Work out the finished part from the listing and answer in its coordinate system (mm). A direction names the side the tool comes from. Give positions to 0.01 mm unless a question says otherwise; leave off trailing zeros. Loops run counter-clockwise (first coordinate to the right, second up) from the corner with the lowest first, then second, coordinate; pieces in that order, holes last. Notation, with made-up numbers: M -6.75,64.5 L -2.75,64.5 A24 ccw -2.75,102.5 Z; hole C 1,19 d7. An arc over 180 degrees is marked long. Use a Markdown table: item, result.
```python
from build123d import *

# Parameters (mm, degrees)
BASE_W              = 40
BASE_H              = 59
EXTRUDE_1_DEPTH     = 2
SKETCH_2_W          = 40
SKETCH_2_H          = 59
SKETCH_2_W_2        = 35
SKETCH_2_H_2        = 54
EXTRUDE_2_DEPTH     = 10
SKETCH_3_R          = 3.25
EXTRUDE_3_DEPTH     = 5
SKETCH_4_R          = 2.9
CUT_EXTRUDE_2_DEPTH = 5
CHAMFER_1_SIZE      = 1.5
CHAMFER_1_SIZE_2    = 5.598076211
SKETCH_6_R          = 1.75
CUT_EXTRUDE_3_DEPTH = 38.896736188
FILLET_1_R          = 5
SKETCH_7_W          = 40
SKETCH_7_H          = 59
SKETCH_7_W_2        = 39
SKETCH_7_H_2        = 58
CUT_EXTRUDE_6_DEPTH = 6
CHAMFER_2_SIZE      = 1
SKETCH_8_W          = 43.293299122
SKETCH_8_H          = 71.249143308
CUT_EXTRUDE_7_DEPTH = 0.1
SKETCH_9_W          = 16
SKETCH_9_H          = 3
CUT_EXTRUDE_8_DEPTH = 64.13297577


with BuildPart() as part:
    # base → Бобышка-Вытянуть1 (new body)
    with BuildSketch(Plane.XY):
        with Locations((-0.540511526, 0)):
            Rectangle(BASE_W, BASE_H)
    extrude(amount=EXTRUDE_1_DEPTH)

    # Эскиз2 → Бобышка-Вытянуть2 (add)
    with BuildSketch(Plane.XY.offset(2)):
        with Locations((-0.540511526, 0)):
            Rectangle(SKETCH_2_W, SKETCH_2_H)
        with Locations((-0.540511526, 0)):
            Rectangle(SKETCH_2_W_2, SKETCH_2_H_2, mode=Mode.SUBTRACT)
    extrude(amount=EXTRUDE_2_DEPTH)

    # Эскиз3 → Бобышка-Вытянуть3 (add)
    with BuildSketch(Plane.XY.offset(2)):
        with Locations((-14.040511526, -23)):
            Circle(SKETCH_3_R)
        with Locations((12.959488474, -23)):
            Circle(SKETCH_3_R)
        with Locations((12.959488474, 23)):
            Circle(SKETCH_3_R)
        with Locations((-14.040511526, 23)):
            Circle(SKETCH_3_R)
    extrude(amount=EXTRUDE_3_DEPTH)

    # Эскиз4 → Вырез-Вытянуть2 (cut)
    with BuildSketch(Plane(origin=(0, 0, 0), x_dir=(-1, 0, 0), z_dir=(0, 0, -1))):
        with Locations((14.040511526, -23)):
            Circle(SKETCH_4_R)
        with Locations((-12.959488474, -23)):
            Circle(SKETCH_4_R)
        with Locations((-12.959488474, 23)):
            Circle(SKETCH_4_R)
        with Locations((14.040511526, 23)):
            Circle(SKETCH_4_R)
    extrude(amount=-CUT_EXTRUDE_2_DEPTH, mode=Mode.SUBTRACT)

    # Фаска1
    # the kernel refuses this chamfer: 5.598076211, 1.5 mm, written as the material it adds along each edge
    with BuildSketch(Plane(origin=(-14.040511526, 23, 2), x_dir=(1, 0, 0), z_dir=(0, -1, 0))) as chamfer_1_piece_1_section:
        Polygon((3.25 + CHAMFER_1_SIZE, 0), (3.25, CHAMFER_1_SIZE_2), (3.25, 0), align=None)
    chamfer_1_piece_1 = revolve(axis=Axis((-14.040511526, 23, 2), (0, 0, 1)), mode=Mode.PRIVATE)
    chamfer_1_piece_1 = split(chamfer_1_piece_1, bisect_by=Plane(origin=(-14.040511526, 23, 7), z_dir=(0, 0, -1)), keep=Keep.TOP, mode=Mode.PRIVATE)
    add(chamfer_1_piece_1)
    with BuildSketch(Plane(origin=(12.959488474, 23, 2), x_dir=(1, 0, 0), z_dir=(0, -1, 0))) as chamfer_1_piece_2_section:
        Polygon((3.25 + CHAMFER_1_SIZE, 0), (3.25, CHAMFER_1_SIZE_2), (3.25, 0), align=None)
    chamfer_1_piece_2 = revolve(axis=Axis((12.959488474, 23, 2), (0, 0, 1)), mode=Mode.PRIVATE)
    chamfer_1_piece_2 = split(chamfer_1_piece_2, bisect_by=Plane(origin=(12.959488474, 23, 7), z_dir=(0, 0, -1)), keep=Keep.TOP, mode=Mode.PRIVATE)
    add(chamfer_1_piece_2)
    with BuildSketch(Plane(origin=(-14.040511526, -23, 2), x_dir=(1, 0, 0), z_dir=(0, -1, 0))) as chamfer_1_piece_3_section:
        Polygon((3.25 + CHAMFER_1_SIZE, 0), (3.25, CHAMFER_1_SIZE_2), (3.25, 0), align=None)
    chamfer_1_piece_3 = revolve(axis=Axis((-14.040511526, -23, 2), (0, 0, 1)), mode=Mode.PRIVATE)
    chamfer_1_piece_3 = split(chamfer_1_piece_3, bisect_by=Plane(origin=(-14.040511526, -23, 7), z_dir=(0, 0, -1)), keep=Keep.TOP, mode=Mode.PRIVATE)
    add(chamfer_1_piece_3)
    with BuildSketch(Plane(origin=(12.959488474, -23, 2), x_dir=(1, 0, 0), z_dir=(0, -1, 0))) as chamfer_1_piece_4_section:
        Polygon((3.25 + CHAMFER_1_SIZE, 0), (3.25, CHAMFER_1_SIZE_2), (3.25, 0), align=None)
    chamfer_1_piece_4 = revolve(axis=Axis((12.959488474, -23, 2), (0, 0, 1)), mode=Mode.PRIVATE)
    chamfer_1_piece_4 = split(chamfer_1_piece_4, bisect_by=Plane(origin=(12.959488474, -23, 7), z_dir=(0, 0, -1)), keep=Keep.TOP, mode=Mode.PRIVATE)
    add(chamfer_1_piece_4)

    # Эскиз6 → Вырез-Вытянуть3 (cut, through all)
    with BuildSketch(Plane(origin=(0, 0, 0), x_dir=(-1, 0, 0), z_dir=(0, 0, -1))):
        with Locations((-12.959488474, 23)):
            Circle(SKETCH_6_R)
        with Locations((14.040511526, 23)):
            Circle(SKETCH_6_R)
        with Locations((14.040511526, -23)):
            Circle(SKETCH_6_R)
        with Locations((-12.959488474, -23)):
            Circle(SKETCH_6_R)
    extrude(amount=-CUT_EXTRUDE_3_DEPTH, mode=Mode.SUBTRACT)

    # Скругление1
    # the kernel refuses this fillet: 5 mm, written as the material it takes off along each edge
    with BuildSketch(Plane(origin=(19.459488474, -42, 0), x_dir=(0, 0, 1), z_dir=(0, 1, 0)), Plane(origin=(-20.540511526, 42, 0), x_dir=(0, 0, 1), z_dir=(0, -1, 0))) as fillet_1_piece_1:
        with BuildLine():
            CenterArc((FILLET_1_R, -FILLET_1_R), FILLET_1_R, 90, 90)
            Line((0, -FILLET_1_R), (0, 0))
            Line((0, 0), (FILLET_1_R, 0))
        make_face()
    extrude(amount=84, mode=Mode.SUBTRACT)

    # Эскиз7 → Вырез-Вытянуть6 (cut)
    with BuildSketch(Plane.XY.offset(12)):
        with Locations((-0.540511526, 0)):
            Rectangle(SKETCH_7_W, SKETCH_7_H)
        with Locations((-0.540511526, 0)):
            Rectangle(SKETCH_7_W_2, SKETCH_7_H_2, mode=Mode.SUBTRACT)
    extrude(amount=-CUT_EXTRUDE_6_DEPTH, mode=Mode.SUBTRACT)

    # Фаска2
    chamfer_2_edges = [part.edges().sort_by_distance(p)[0] for p in [
        (-20.040511526, 29, 9),
        (-20.040511526, -29, 9),
        (18.959488474, -29, 9),
        (18.959488474, 29, 9),
    ]]
    chamfer(chamfer_2_edges, length=CHAMFER_2_SIZE)

    # Эскиз8 → Вырез-Вытянуть7 (cut)
    with BuildSketch(Plane.XY.offset(12)):
        with Locations((-1.042207714, -0.462672782)):
            Rectangle(SKETCH_8_W, SKETCH_8_H)
    extrude(amount=-CUT_EXTRUDE_7_DEPTH, mode=Mode.SUBTRACT)

    # Эскиз9 → Вырез-Вытянуть8 (cut, through all)
    with BuildSketch(Plane(origin=(0, 29, 0), x_dir=(1, 0, 0), z_dir=(0, 1, 0))):
        with Locations((-2.179108085, -10.4)):
            Rectangle(SKETCH_9_W, SKETCH_9_H)
    extrude(amount=-CUT_EXTRUDE_8_DEPTH, mode=Mode.SUBTRACT)


solid = part.part
```
(1) Given P1, Ø3, axis at y = 12, z = 9, coming from the -X side; P2, Ø5, axis at x = -3, z = 9, coming from the +Y side; P3, Ø1, axis at x = -5.5, y = -28, coming from the +Z side, each flat-ended and moving along its own axis, determine where each tip first touches the part or whether it passes through.
Entries:
| item | result |
|---|---|
| P1 | stops at x = -20.04 |
| P2 | stops at y = 29 |
| P3 | stops at z = 8.9 |
(2) Which of the six approach directions +Z, -Z, +X, -X, +Y, -Y give full straight-line access (tool end or side, diameter ignored) to faces 5 (the cylindrical face through (11.62, 20.43, 2.46)), 6 (the flat face through (18.959, 0, 9)), 7 (the flat face through (-1, -29, 8))?
Entries:
| item | result |
|---|---|
| face 5 | -Z |
| face 6 | +Z, +X, +Y, -Y |
| face 7 | +Z, +X, -X, -Y |
(3) Consider probe 1 along X at (y, z) = (-10.5, 8.75); probe 2 along Y at (x, z) = (-12, 2.25); probe 3 along X at (y, z) = (26, 6.25). Determine where each line is inside the solid, lowest interval first. Write a range as [from, to].
Entries:
| item | result |
|---|---|
| probe 1 | x = [-20.04, -18.04], [16.96, 18.96] |
| probe 2 | y = [-29.5, -25.06], [-20.94, -18.78], [18.78, 20.94], [25.06, 29.5] |
| probe 3 | x = [-20.04, -18.04], [-16.05, -12.03], [10.95, 14.97], [16.96, 18.96] |
(4) A cutting plane is placed at B-B (y = -23). Count the separate pieces of the cut face and the enclosed holes in it, and give its area (3 significant figures).
Entries:
| item | result |
|---|---|
| separate pieces | 3 |
| enclosed holes | 0 |
| area | 121 mm² |
(5) A cutting plane is placed at A-A (z = 7.75). Write down the section's boundary in (x, y), and give its area (3 significant figures).
Entries:
| item | result |
|---|---|
| outline | M -20.04,-28 L -19.04,-29 L 17.96,-29 L 18.96,-28 L 18.96,28 L 17.96,29 L -19.04,29 L -20.04,28 Z; hole M -18.04,-27 L 16.96,-27 L 16.96,27 L -18.04,27 Z |
| area | 370 mm² |
(6) The mould has two halves that part along Y. Classify faces 1 (the flat face through (-18.041, 0, 7)), 2 (the cylindrical face through (-13.813, -21.265, 5.986)), 3 (the flat face through (-1, -29.5, 3)), 4 (the flat face through (-10.179, 28, 10)): released by +Y, released by -Y, zero draft, split by the parting line, or undercut.
Entries:
| item | result |
|---|---|
| face 1 | undercut |
| face 2 | undercut |
| face 3 | released by -Y |
| face 4 | zero draft |
(7) A cutting plane is placed at C-C (x = -6). Write down the section's boundary in (y, z).
Entries:
| item | result |
|---|---|
| outline | M -29.5,0 L 29.5,0 L 29.5,6 L 29,6 L 29,8.9 L 27,8.9 L 27,2 L -27,2 L -27,8.9 L -29,8.9 L -29,6 L -29.5,6 Z |
